from build123d import *

# Parameters (mm, degrees)
BR_EXTRUDE_DEPTH      = 97.5
BR_EXTRUDE_DEPTH_BACK = 52.5


with BuildPart() as part:
    # Sketch2 → BR_Extrude (new body, two sides)
    with BuildSketch(Plane(origin=(0, 0, 0), x_dir=(0, 0, -1), z_dir=(1, 0, 0))) as br_extrude_sk:
        with BuildLine():
            Line((-10.05, 11.676345597), (-10.05, 16.5))
            Line((-10.05, 16.5), (-5, 16.5))
            Line((-5, 16.5), (-5, 21))
            Line((-5, 21), (-5.8, 21))
            Line((-5.8, 21), (-5.8, 22.5))
            Line((-5.8, 22.5), (-19.5, 22.5))
            ThreePointArc((-19.5, 22.5), (-21.621320344, 21.621320344), (-22.5, 19.5))
            Line((-22.5, 19.5), (-22.5, 5.8))
            Line((-22.5, 5.8), (-21, 5.8))
            Line((-21, 5.8), (-21, 5))
            Line((-21, 5), (-16.5, 5))
            Line((-16.5, 5), (-16.5, 10.05))
            Line((-16.5, 10.05), (-11.676345597, 10.05))
            Line((-11.676345597, 10.05), (-6.411275155, 4.784929559))
            ThreePointArc((-6.411275155, 4.784929559), (-8, 0), (-6.411275155, -4.784929559))
            Line((-6.411275155, -4.784929559), (-11.676345597, -10.05))
            Line((-11.676345597, -10.05), (-16.5, -10.05))
            Line((-16.5, -10.05), (-16.5, -5))
            Line((-16.5, -5), (-21, -5))
            Line((-21, -5), (-21, -5.8))
            Line((-21, -5.8), (-22.5, -5.8))
            Line((-22.5, -5.8), (-22.5, -19.5))
            ThreePointArc((-22.5, -19.5), (-21.621320344, -21.621320344), (-19.5, -22.5))
            Line((-19.5, -22.5), (-5.8, -22.5))
            Line((-5.8, -22.5), (-5.8, -21))
            Line((-5.8, -21), (-5, -21))
            Line((-5, -21), (-5, -16.5))
            Line((-5, -16.5), (-10.05, -16.5))
            Line((-10.05, -16.5), (-10.05, -11.676345597))
            Line((-10.05, -11.676345597), (-4.784929559, -6.411275155))
            ThreePointArc((-4.784929559, -6.411275155), (0, -8), (4.784929559, -6.411275155))
            Line((4.784929559, -6.411275155), (10.05, -11.676345597))
            Line((10.05, -11.676345597), (10.05, -16.5))
            Line((10.05, -16.5), (5, -16.5))
            Line((5, -16.5), (5, -21))
            Line((5, -21), (5.8, -21))
            Line((5.8, -21), (5.8, -22.5))
            Line((5.8, -22.5), (19.5, -22.5))
            ThreePointArc((19.5, -22.5), (21.621320344, -21.621320344), (22.5, -19.5))
            Line((22.5, -19.5), (22.5, -5.8))
            Line((22.5, -5.8), (21, -5.8))
            Line((21, -5.8), (21, -5))
            Line((21, -5), (16.5, -5))
            Line((16.5, -5), (16.5, -10.05))
            Line((16.5, -10.05), (11.676345597, -10.05))
            Line((11.676345597, -10.05), (6.411275155, -4.784929559))
            ThreePointArc((6.411275155, -4.784929559), (8, 0), (6.411275155, 4.784929559))
            Line((6.411275155, 4.784929559), (11.676345597, 10.05))
            Line((11.676345597, 10.05), (16.5, 10.05))
            Line((16.5, 10.05), (16.5, 5))
            Line((16.5, 5), (21, 5))
            Line((21, 5), (21, 5.8))
            Line((21, 5.8), (22.5, 5.8))
            Line((22.5, 5.8), (22.5, 19.5))
            ThreePointArc((22.5, 19.5), (21.621320344, 21.621320344), (19.5, 22.5))
            Line((19.5, 22.5), (5.8, 22.5))
            Line((5.8, 22.5), (5.8, 21))
            Line((5.8, 21), (5, 21))
            Line((5, 21), (5, 16.5))
            Line((5, 16.5), (10.05, 16.5))
            Line((10.05, 16.5), (10.05, 11.676345597))
            Line((10.05, 11.676345597), (4.784929559, 6.411275155))
            ThreePointArc((4.784929559, 6.411275155), (0, 8), (-4.784929559, 6.411275155))
            Line((-4.784929559, 6.411275155), (-10.05, 11.676345597))
        make_face()
        with BuildLine():
            Line((11.55, 11.55), (11.55, 18))
            Line((11.55, 18), (7.5, 18))
            Line((7.5, 18), (7.5, 21))
            Line((7.5, 21), (18.5, 21))
            ThreePointArc((18.5, 21), (20.267766953, 20.267766953), (21, 18.5))
            Line((21, 18.5), (21, 7.5))
            Line((21, 7.5), (18, 7.5))
            Line((18, 7.5), (18, 11.55))
            Line((18, 11.55), (11.55, 11.55))
        make_face(mode=Mode.SUBTRACT)
        with BuildLine():
            Line((11.55, -11.55), (18, -11.55))
            Line((18, -11.55), (18, -7.5))
            Line((18, -7.5), (21, -7.5))
            Line((21, -7.5), (21, -18.5))
            ThreePointArc((21, -18.5), (20.267766953, -20.267766953), (18.5, -21))
            Line((18.5, -21), (7.5, -21))
            Line((7.5, -21), (7.5, -18))
            Line((7.5, -18), (11.55, -18))
            Line((11.55, -18), (11.55, -11.55))
        make_face(mode=Mode.SUBTRACT)
        with BuildLine():
            Line((-11.55, 11.55), (-18, 11.55))
            Line((-18, 11.55), (-18, 7.5))
            Line((-18, 7.5), (-21, 7.5))
            Line((-21, 7.5), (-21, 18.5))
            ThreePointArc((-21, 18.5), (-20.267766953, 20.267766953), (-18.5, 21))
            Line((-18.5, 21), (-7.5, 21))
            Line((-7.5, 21), (-7.5, 18))
            Line((-7.5, 18), (-11.55, 18))
            Line((-11.55, 18), (-11.55, 11.55))
        make_face(mode=Mode.SUBTRACT)
        with BuildLine():
            Line((-11.55, -11.55), (-11.55, -18))
            Line((-11.55, -18), (-7.5, -18))
            Line((-7.5, -18), (-7.5, -21))
            Line((-7.5, -21), (-18.5, -21))
            ThreePointArc((-18.5, -21), (-20.267766953, -20.267766953), (-21, -18.5))
            Line((-21, -18.5), (-21, -7.5))
            Line((-21, -7.5), (-18, -7.5))
            Line((-18, -7.5), (-18, -11.55))
            Line((-18, -11.55), (-11.55, -11.55))
        make_face(mode=Mode.SUBTRACT)
        with BuildLine():
            Line((-6.007327293, -1.059253884), (-4.924038765, -0.868240888))
            ThreePointArc((-4.924038765, -0.868240888), (-5, 0), (-4.924038765, 0.868240888))
            Line((-4.924038765, 0.868240888), (-6.007327293, 1.059253884))
            ThreePointArc((-6.007327293, 1.059253884), (-5.635665148, 2.334368937), (-4.99682747, 3.498816262))
            Line((-4.99682747, 3.498816262), (-4.095760221, 2.867882182))
            ThreePointArc((-4.095760221, 2.867882182), (-3.535533906, 3.535533906), (-2.867882182, 4.095760221))
            Line((-2.867882182, 4.095760221), (-3.498816262, 4.99682747))
            ThreePointArc((-3.498816262, 4.99682747), (-2.334368937, 5.635665148), (-1.059253884, 6.007327293))
            Line((-1.059253884, 6.007327293), (-0.868240888, 4.924038765))
            ThreePointArc((-0.868240888, 4.924038765), (0, 5), (0.868240888, 4.924038765))
            Line((0.868240888, 4.924038765), (1.059253884, 6.007327293))
            ThreePointArc((1.059253884, 6.007327293), (2.334368937, 5.635665148), (3.498816262, 4.99682747))
            Line((3.498816262, 4.99682747), (2.867882182, 4.095760221))
            ThreePointArc((2.867882182, 4.095760221), (3.535533906, 3.535533906), (4.095760221, 2.867882182))
            Line((4.095760221, 2.867882182), (4.99682747, 3.498816262))
            ThreePointArc((4.99682747, 3.498816262), (5.635665148, 2.334368937), (6.007327293, 1.059253884))
            Line((6.007327293, 1.059253884), (4.924038765, 0.868240888))
            ThreePointArc((4.924038765, 0.868240888), (5, 0), (4.924038765, -0.868240888))
            Line((4.924038765, -0.868240888), (6.007327293, -1.059253884))
            ThreePointArc((6.007327293, -1.059253884), (5.635665148, -2.334368937), (4.99682747, -3.498816262))
            Line((4.99682747, -3.498816262), (4.095760221, -2.867882182))
            ThreePointArc((4.095760221, -2.867882182), (3.535533906, -3.535533906), (2.867882182, -4.095760221))
            Line((2.867882182, -4.095760221), (3.498816262, -4.99682747))
            ThreePointArc((3.498816262, -4.99682747), (2.334368937, -5.635665148), (1.059253884, -6.007327293))
            Line((1.059253884, -6.007327293), (0.868240888, -4.924038765))
            ThreePointArc((0.868240888, -4.924038765), (0, -5), (-0.868240888, -4.924038765))
            Line((-0.868240888, -4.924038765), (-1.059253884, -6.007327293))
            ThreePointArc((-1.059253884, -6.007327293), (-2.334368937, -5.635665148), (-3.498816262, -4.99682747))
            Line((-3.498816262, -4.99682747), (-2.867882182, -4.095760221))
            ThreePointArc((-2.867882182, -4.095760221), (-3.535533906, -3.535533906), (-4.095760221, -2.867882182))
            Line((-4.095760221, -2.867882182), (-4.99682747, -3.498816262))
            ThreePointArc((-4.99682747, -3.498816262), (-5.635665148, -2.334368937), (-6.007327293, -1.059253884))
        make_face(mode=Mode.SUBTRACT)
    extrude(amount=BR_EXTRUDE_DEPTH)
    extrude(br_extrude_sk.sketch, amount=-BR_EXTRUDE_DEPTH_BACK)


solid = part.part
Here's how the part is built. I have some questions about the finished solid (model axes, mm). A direction names the side the tool comes from. Give positions to 0.01 mm unless a question says otherwise; leave off trailing zeros. Order: outer loops, then holes, each group sorted by start corner. A loop starts at its lowest first (then second) coordinate and runs counter-clockwise, first axis right, second up. Notation, with made-up numbers: M 30.25,76.5 L 42.25,76.5 A23 ccw 42.25,107.5 Z; hole C 48.25,-39 d11. An arc over 180 degrees is marked long. Answer as a JSON object with one key per item and string values. Group by question number.
1) We'd pull the mould along Y, two halves only. Please class faces 5 (the flat face through (24, 13, 21)), 6 (the flat face through (97.5, 2, 7)), 7 (the flat face through (24, -22.5, -13)): pulls with the +Y half, pulls with the -Y half, needs draft (parallel to the pull), parting line crosses it, or undercut.
2) Suppose I cut it at B-B, the plane x = 6.5. Count the separate pieces of the cut face and the enclosed holes in it, plus the area to 3 significant figures.
3) Suppose I cut it at A-A, the plane y = 14.5. Write out the boundary of the cut face in (x, z), plus the area to 3 significant figures.
4) On a 3-axis mill with a long thin cutter (end or side, diameter ignored), from which of +Z, -Z, +X, -X, +Y, -Y can I reach the whole of each face in a straight line? I mean faces 1 (the flat face through (24, -5, 19)), 2 (the flat face through (24, -13, -21)), 3 (the flat face through (24, 19, 5)), 4 (the flat face through (24, -5, -19)). Say none if no direction works.
5) Please list where these lines run through material, in increasing order: L1, parallel to Z at x = 61, y = 13; L2, parallel to Z at x = 16.5, y = -18.5. Write a range as [from, to].
6) I'm going to push flat-ended pins straight in: pin 1 Ø1.2 at (x, y) = (35.5, 22) entering from -Z; pin 2 Ø5 at (x, y) = (61.5, 0) entering from -Z; pin 3 Ø1.5 at (x, z) = (0, -4) entering from +Y. Where does each tip first touch, or does it pass through?
Results found:
{
 "1": {"face 5": "undercut", "face 6": "needs draft", "face 7": "pulls with the -Y half"},
 "2": {"separate pieces": "1", "enclosed holes": "5", "area": "560 mm²"},
 "3": {"outline": "M -52.5,-22.5 L 97.5,-22.5 L 97.5,-21 L -52.5,-21 Z; M -52.5,-11.55 L 97.5,-11.55 L 97.5,-10.05 L -52.5,-10.05 Z; M -52.5,10.05 L 97.5,10.05 L 97.5,11.55 L -52.5,11.55 Z; M -52.5,21 L 97.5,21 L 97.5,22.5 L -52.5,22.5 Z", "area": "900 mm²"},
 "4": {"face 1": "+Z, +X, -X", "face 2": "+X, -X", "face 3": "+X, -X, +Y", "face 4": "-Z, +X, -X"},
 "5": {"L1": "[-22.5, -21], [-11.55, -10.05], [10.05, 11.55], [21, 22.5]", "L2": "[-22.5, -21], [-7.5, -5], [5, 7.5], [21, 22.5]"},
 "6": {"pin 1": "z = -21.82", "pin 2": "z = -8", "pin 3": "y = 7.31"}
}
